The listing builds one solid part. Answer for the finished solid, in the listing's coordinates (mm). Coordinates: 2 decimals unless noted, no trailing zeros. Order: outer loops, then holes, each group sorted by start corner. A loop starts at its lowest first (then second) coordinate and runs counter-clockwise, first axis right, second up.
from build123d import *

# Parameters (mm, degrees)
SKETCH4_W           = 45.72
SKETCH4_H           = 38.1
BOSS_EXTRUDE1_DEPTH = 2.54
SKETCH5_R           = 1.65
SKETCH5_R_2         = 1.32
CUT_EXTRUDE1_DEPTH  = 2.54


with BuildPart() as part:
    # Sketch4 → Boss-Extrude1 (new body)
    with BuildSketch(Plane(origin=(0, 0, 0), x_dir=(1, 0, 0), z_dir=(0, 1, 0))):
        with Locations((22.86, 19.05)):
            Rectangle(SKETCH4_W, SKETCH4_H)
    extrude(amount=BOSS_EXTRUDE1_DEPTH)

    # Sketch5 → Cut-Extrude1 (cut)
    with BuildSketch(Plane.XZ):
        with Locations((3.3655, -24.892)):
            Circle(SKETCH5_R)
        with Locations((3.3655, -34.892)):
            Circle(SKETCH5_R)
        with Locations((10.668, -4.6228)):
            Circle(SKETCH5_R_2)
        with Locations((10.668, -32.5628)):
            Circle(SKETCH5_R_2)
        with Locations((41.148, -4.6228)):
            Circle(SKETCH5_R_2)
        with Locations((41.148, -32.5628)):
            Circle(SKETCH5_R_2)
    extrude(amount=-CUT_EXTRUDE1_DEPTH, mode=Mode.SUBTRACT)


solid = part.part
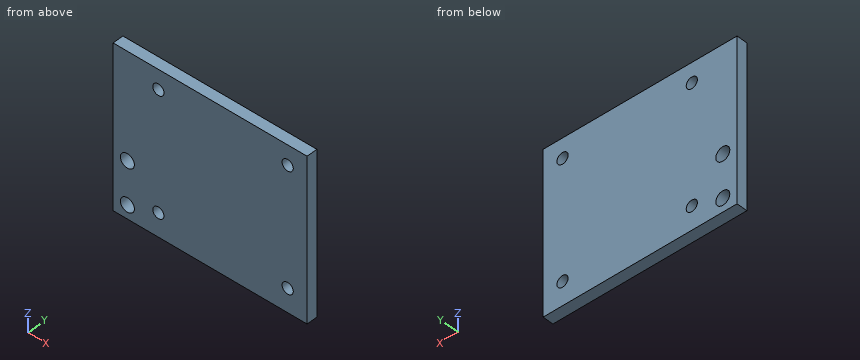
(1) Find section C-C on x = 3. Determine the outline of the cut face in (y, z), then the cut area to 3 significant figures.
(2) Find the intervals of material crossed by probe 1 along Z at (x, y) = (2.5, 1.5); probe 2 along X at (y, z) = (2.3, -4); probe 3 along X at (y, z) = (2.2, -33), in increasing order.
(3) Find section B-B on y = 1.7. Determine the outline of the cut face in (x, z).
(4) Given pin 1 Ø1.6 at (x, z) = (41.15, -32.56) entering from -Y, flat-ended and moving along its own axis, determine where the tip first touches the part or whether it passes through.
(5) Find section A-A on x = 41. Determine the outline of the cut face in (y, z).
Resolved:
1. outline: (0, -38.1) - (2.54, -38.1) - (2.54, -36.5) - (0, -36.5) - close; (0, -33.28) - (2.54, -33.28) - (2.54, -26.5) - (0, -26.5) - close; (0, -23.28) - (2.54, -23.28) - (2.54, 0) - (0, 0) - close
1. area: 80.4 mm2
2. probe 1: z = -38.1 to -36.3, -33.49 to -26.3, -23.49 to 0
2. probe 2: x = 0 to 9.5, 11.83 to 39.98, 42.31 to 45.72
2. probe 3: x = 0 to 9.42, 11.91 to 39.9, 42.39 to 45.72
3. outline: (0, -38.1) - (45.72, -38.1) - (45.72, 0) - (0, 0) - close; hole circle Ø3.3 at (3.37, -34.89); hole circle Ø3.3 at (3.37, -24.89); hole circle Ø2.64 at (10.67, -32.56); hole circle Ø2.64 at (10.67, -4.62); hole circle Ø2.64 at (41.15, -32.56); hole circle Ø2.64 at (41.15, -4.62)
4. pin 1: passes through
5. outline: (0, -38.1) - (2.54, -38.1) - (2.54, -33.87) - (0, -33.87) - close; (0, -31.25) - (2.54, -31.25) - (2.54, -5.93) - (0, -5.93) - close; (0, -3.31) - (2.54, -3.31) - (2.54, 0) - (0, 0) - close
